Check sheet for the modelled part. Datum: model origin and axes. Units: mm. Face numbers are marked on the shaded views. Coordinates: 2 decimals unless noted, no trailing zeros. Loops run counter-clockwise (first coordinate to the right, second up) from the corner with the lowest first, then second, coordinate; pieces in that order, holes last.
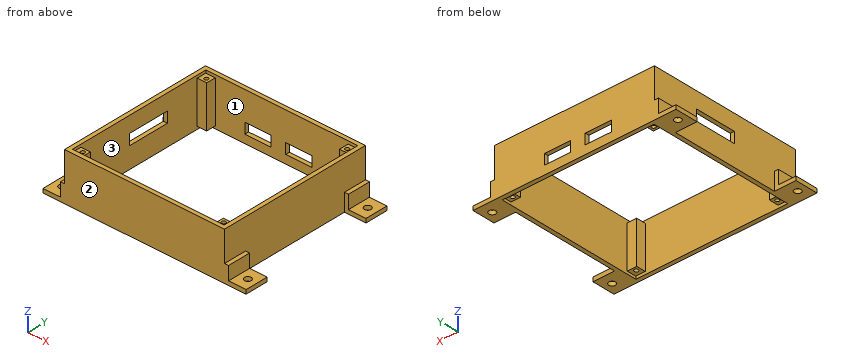
```python
from build123d import *

# Parameters (mm, degrees)
F0_W      = 118.5
F0_H      = 114
F0_W_2    = 112.5
F0_H_2    = 108
F1_DEPTH  = 35.36
F3_START  = -2
F2_W      = 7
F2_H      = 7
F3_DEPTH  = 31.36
F4_R      = 1.45
F5_DEPTH  = 33.361
F6_W      = 30.51
F6_H      = 8
F7_DEPTH  = 3
F8_W      = 19.4
F8_H      = 7.7
F9_DEPTH  = 3
F11_DEPTH = 114
F13_DEPTH = 114
F15_W     = 16
F15_H     = 80
F16_DEPTH = 35.361
F17_W     = 16
F17_H     = 80
F18_DEPTH = 35.361
F19_R     = 2.5
F20_DEPTH = 3.001


# Not quite as in the source:
# - a feature names something its author has since deleted; it is built from what else it names


with BuildPart() as f1:
    # F0 (on Top) → F1 (new body)
    with BuildSketch(Plane.XY):
        with Locations((56.25, 54)):
            Rectangle(F0_W, F0_H)
        with Locations((56.25, 54)):
            Rectangle(F0_W_2, F0_H_2, mode=Mode.SUBTRACT)
    extrude(amount=F1_DEPTH)

    # F2 (on face) → F3 (join)
    with BuildSketch(Plane.XY.offset(35.36).offset(F3_START)):
        with Locations((3.5, 104.5)):
            Rectangle(F2_W, F2_H)
        with Locations((109, 104.5)):
            Rectangle(F2_W, F2_H)
        with Locations((109, 3.5)):
            Rectangle(F2_W, F2_H)
        with Locations((3.5, 3.5)):
            Rectangle(F2_W, F2_H)
    extrude(amount=-F3_DEPTH)

    # F4 (on face) → F5 (cut, through all)
    with BuildSketch(Plane.XY.offset(33.36)):
        with Locations((4, 104)):
            Circle(F4_R)
        with Locations((108.5, 104)):
            Circle(F4_R)
        with Locations((4, 4)):
            Circle(F4_R)
        with Locations((108.5, 4)):
            Circle(F4_R)
    extrude(amount=-F5_DEPTH, mode=Mode.SUBTRACT)

    # F6 (on face) → F7 (cut, through all)
    with BuildSketch(Plane(origin=(-3, 0, 0), x_dir=(0, -1, 0), z_dir=(-1, 0, 0))):
        with Locations((-61.615, 19.54)):
            Rectangle(F6_W, F6_H)
    extrude(amount=-F7_DEPTH, mode=Mode.SUBTRACT)

    # F8 (on face) → F9 (cut)
    with BuildSketch(Plane(origin=(0, 111, 0), x_dir=(-1, 0, 0), z_dir=(0, 1, 0))):
        with Locations((-68.83, 10.11)):
            Rectangle(F8_W, F8_H)
        with Locations((-38.62, 10.11)):
            Rectangle(F8_W, F8_H)
    extrude(amount=-F9_DEPTH, mode=Mode.SUBTRACT)

    # F10 (on face) → F11 (join)
    with BuildSketch(Plane.XZ.offset(3)):
        Polygon((-6, 3), (-19, 3), (-19, 0), (-3, 0), (-3, 13), (-6, 13), align=None)
    extrude(amount=-F11_DEPTH)

    # F12 (on face) → F13 (join)
    with BuildSketch(Plane.XZ.offset(3)):
        Polygon((118.5, 13), (115.5, 13), (115.5, 0), (131.5, 0), (131.5, 3), (118.5, 3), align=None)
    extrude(amount=-F13_DEPTH)

    # F15 (on face) → F16 (cut, through all)
    with BuildSketch(Plane(origin=(0, 0, 0), x_dir=(1, 0, 0), z_dir=(0, 0, -1))):
        with Locations((-11, -54)):
            Rectangle(F15_W, F15_H)
    extrude(amount=-F16_DEPTH, mode=Mode.SUBTRACT)

    # F17 (on face) → F18 (cut, through all)
    with BuildSketch(Plane(origin=(0, 0, 0), x_dir=(1, 0, 0), z_dir=(0, 0, -1))):
        with Locations((123.5, -54)):
            Rectangle(F17_W, F17_H)
    extrude(amount=-F18_DEPTH, mode=Mode.SUBTRACT)

    # F19 (on face) → F20 (cut, through all)
    with BuildSketch(Plane.XY.offset(3)):
        with Locations((-12.5, 102.5)):
            Circle(F19_R)
        with Locations((125, 102.5)):
            Circle(F19_R)
        with Locations((125, 5.5)):
            Circle(F19_R)
        with Locations((-12.5, 5.5)):
            Circle(F19_R)
    extrude(amount=-F20_DEPTH, mode=Mode.SUBTRACT)


solid = f1.part
```
1) Section check C-C on y = 36. Enter the section's corners in (x, z).
Answer sheet:
outline: (-3, 0) - (0, 0) - (0, 35.36) - (-3, 35.36) - close; (112.5, 0) - (115.5, 0) - (115.5, 35.36) - (112.5, 35.36) - close
2) Section check B-B on z = 19. Enter the section's corners in (x, y), plus the area to 3 significant figures.
Answer sheet:
outline: (-3, -3) - (115.5, -3) - (115.5, 111) - (-3, 111) - (-3, 76.87) - (0, 76.87) - (0, 101) - (7, 101) - (7, 108) - (105.5, 108) - (105.5, 101) - (112.5, 101) - (112.5, 7) - (105.5, 7) - (105.5, 0) - (7, 0) - (7, 7) - (0, 7) - (0, 46.36) - (-3, 46.36) - close; hole circle Ø2.9 at (4, 4); hole circle Ø2.9 at (4, 104); hole circle Ø2.9 at (108.5, 4); hole circle Ø2.9 at (108.5, 104)
area: 1,440 mm2
3) Depth check by flat-ended pin: pin 1 (3.5 mm diameter, centred on x = 108.5, y = 5, fed in from -Z); pin 2 (3.5 mm diameter, centred on y = 104, z = 21, fed in from -X); pin 3 (1.5 mm diameter, centred on y = 109, z = 9, fed in from -X). Enter the tip coordinate at first touch or a pass-through.
Answer sheet:
pin 1: stops at z = 2
pin 2: stops at x = -3
pin 3: stops at x = -6
4) Section check A-A on x = 125. Enter the section's corners in (y, z).
Answer sheet:
outline: (-3, 0) - (3, 0) - (3, 3) - (-3, 3) - close; (8, 0) - (14, 0) - (14, 3) - (8, 3) - close; (94, 0) - (100, 0) - (100, 3) - (94, 3) - close; (105, 0) - (111, 0) - (111, 3) - (105, 3) - close
5) Scan lines: line 1 (Y direction, x = -12.5, z = 1.4); line 2 (Y direction, x = 4, z = 25); line 3 (X direction, y = 35.5, z = 3.5). Record each from-to range of solid material in increasing order.
Answer sheet:
line 1: y = -3 to 3, 8 to 14, 94 to 100, 105 to 111
line 2: y = -3 to 2.55, 5.45 to 7, 101 to 102.55, 105.45 to 111
line 3: x = -3 to 0, 112.5 to 115.5
6) Section check D-D on x = 73.5. Enter the section's corners in (y, z), plus the area to 3 significant figures.
Answer sheet:
outline: (-3, 0) - (0, 0) - (0, 35.36) - (-3, 35.36) - close; (108, 0) - (111, 0) - (111, 6.26) - (108, 6.26) - close; (108, 13.96) - (111, 13.96) - (111, 35.36) - (108, 35.36) - close
area: 189 mm2
7) Mould release check, pull along X, two halves, no side actions. Record for the marked faces 1, 2 and 3: +X half, -X half, draft (parallel to the pull), parting line (faces both ways), or undercut.
Answer sheet:
face 1: undercut
face 2: draft
face 3: undercut
